Could you check a few things on this model? Use its own coordinates, in mm. A direction names the side the tool comes from. Give positions to 0.01 mm unless a question says otherwise; leave off trailing zeros. Order: outer loops, then holes, each group sorted by start corner. A loop starts at its lowest first (then second) coordinate and runs counter-clockwise, first axis right, second up. Notation, with made-up numbers: (4, 75) -> (46, 75) arc R11 cw to (46, 93) -> close; hole circle Ø1 at (30.25, 60.25). An arc over 180 degrees is marked (long way). Answer as CSV lines item,"result". Start each with the question number.
(1) I want a section at A-A (z = -29). Please give me the cut outline in (x, y), plus the area to 3 significant figures.
(2) We'd pull the mould along Z, two halves only. Please class faces 5 (the face through (8.71, -12.52, 63.22)), 6 (the face through (-82.165, -13, -46)), 7 (the face through (-12.165, -13, 20)), 8 (the face through (10, -13, 88.043)): released by +Z, released by -Z, zero draft, split by the parting line, or undercut.
(3) I want a section at D-D (z = 51). Please give me the cut outline in (x, y), plus the area to 3 significant figures.
(4) I want a section at C-C (y = -23). Give the number of separate pieces and of enclosed holes in the cut face, plus the area to 3 significant figures.
(5) I want a section at B-B (x = 8.5). Please give me the cut outline in (y, z).
(6) Will these pins go through, and if not, where does the flat tip stop? pin 1 Ø1.5 at (y, z) = (-13, 28) entering from -X; pin 2 Ø9 at (x, z) = (30.33, 70.54) entering from +Y; pin 3 Ø10 at (y, z) = (-3.5, 44) entering from -X; pin 4 Ø7.5 at (y, z) = (-17.5, -59.5) entering from +X.
(7) I need wall thicknesses on L1, parallel to Z at x = -44, y = -12; L2, parallel to Z at x = -11, y = -2.25; L3, parallel to Z at x = -13, y = -7. Which ranges of each line are inside material? Lowest first, please.
(8) On a 3-axis mill with a long thin cutter (end or side, diameter ignored), from which of +Z, -Z, +X, -X, +Y, -Y can I reach the whole of each face in a straight line? I mean faces 1 (the face through (-36.29, -12.52, 63.22)), 2 (the face through (-49.665, -13, 60)), 3 (the face through (-47, -13, 9.231)), 4 (the face through (56, -13, 15.543)). Say none if no direction works.
```python
from build123d import *

# Parameters (mm, degrees)
F0_R     = 7.5
F0_R_2   = 12.5
F1_DEPTH = 25.4


with BuildPart() as f1:
    # F0 (on Front) → F1 (new body)
    with BuildSketch(Plane.XZ):
        Polygon((-12.1652076736, 30.5430293083), (-12.1652076736, 9.2314934358), (45.3347923264, 9.2314934358), (45.3347923264, 15.5430293083), (67.8347923264, 15.5430293083), (67.8347923264, 70.5430293083), (67.8347923264, 88.0430293083), (-49.6652076736, 88.0430293083), (-49.6652076736, 30.5430293083), align=None)
        with Locations((-34.6652076736, 70.5430293083)):
            Circle(F0_R, mode=Mode.SUBTRACT)
        with Locations((-9.6652076736, 70.5430293083)):
            Circle(F0_R, mode=Mode.SUBTRACT)
        with Locations((10.3347923264, 70.5430293083)):
            Circle(F0_R, mode=Mode.SUBTRACT)
        with Locations((30.3347923264, 70.5430293083)):
            Circle(F0_R, mode=Mode.SUBTRACT)
        with Locations((50.3347923264, 70.5430293083)):
            Circle(F0_R, mode=Mode.SUBTRACT)
        Polygon((-12.1652076736, 9.2314934358), (-82.1652076736, 9.2314934358), (-82.1652076736, -38.2685065642), (-82.1652076736, -63.2685065642), (-82.1652076736, -88.2685065642), (-82.1652076736, -103.2685065642), (-62.1652076736, -103.2685065642), (-37.1652076736, -103.2685065642), (-12.1652076736, -103.2685065642), (45.3347923264, -103.2685065642), (45.3347923264, 9.2314934358), align=None)
        with Locations((-62.1652076736, -88.2685065642)):
            Circle(F0_R_2, mode=Mode.SUBTRACT)
        with Locations((-37.1652076736, -63.2685065642)):
            Circle(F0_R_2, mode=Mode.SUBTRACT)
        with Locations((-12.1652076736, -38.2685065642)):
            Circle(F0_R_2, mode=Mode.SUBTRACT)
    extrude(amount=F1_DEPTH)


solid = f1.part
```
Final values:
1,outline,"(-82.17, -25.4) -> (-20.55, -25.4) -> (-20.55, 0) -> (-82.17, 0) -> close; (-3.78, -25.4) -> (45.33, -25.4) -> (45.33, 0) -> (-3.78, 0) -> close"
1,area,"2,810 mm²"
2,face 5,"undercut"
2,face 6,"zero draft"
2,face 7,"undercut"
2,face 8,"released by +Z"
3,outline,"(-49.67, -25.4) -> (67.83, -25.4) -> (67.83, 0) -> (-49.67, 0) -> close"
3,area,"2,980 mm²"
4,separate pieces,"1"
4,enclosed holes,"8"
4,area,"20,300 mm²"
5,outline,"(-25.4, -103.27) -> (0, -103.27) -> (0, 63.27) -> (-25.4, 63.27) -> close; (-25.4, 77.82) -> (0, 77.82) -> (0, 88.04) -> (-25.4, 88.04) -> close"
6,pin 1,"x = -12.17"
6,pin 2,"through"
6,pin 3,"x = -49.67"
6,pin 4,"x = 45.33"
7,L1,"-103.27 to -73.73, -52.8 to 9.23, 30.54 to 88.04"
7,L2,"-103.27 to -50.71, -25.82 to 63.16, 77.92 to 88.04"
7,L3,"-103.27 to -50.74, -25.8 to 9.23, 30.54 to 63.83, 77.26 to 88.04"
8,face 1,"+Y, -Y"
8,face 2,"+Z, -X, +Y, -Y"
8,face 3,"-X, +Y, -Y"
8,face 4,"-Z, +X, +Y, -Y"
